Read the model definition and answer for the solid it produces. Units are mm, in the model's axes. A direction names the side the tool comes from. Give positions to 0.01 mm unless a question says otherwise; leave off trailing zeros. Loops run counter-clockwise (first coordinate to the right, second up) from the corner with the lowest first, then second, coordinate; pieces in that order, holes last. Notation, with made-up numbers: (25.5, 58.25) - (47.5, 58.25) arc R5 cw to (47.5, 62.25) - close; hole circle Ø4 at (14, 73). An arc over 180 degrees is marked (long way). Put each result on its own line as item: value. Start each with the question number.
1. A cutting plane is placed at A-A, the plane y = 10.5. Determine the outline of the cut face in (x, z) (3 decimals).
2. A cutting plane is placed at C-C, the plane x = 25.4. Determine the outline of the cut face in (y, z) (1 decimal), plus the area to 3 significant figures.
3. A cutting plane is placed at B-B, the plane z = 253.5. Determine the outline of the cut face in (x, y) (3 decimals), plus the area to 3 significant figures.
4. For faces 1 (the flat face through (25, 23, 0)), 2 (the cylindrical face through (22.3, 23.83, 536.71)), 3 (the flat face through (26, 22.225, 299)), determine the directions among +Z, -Z, +X, -X, +Y, -Y from which every point of the face is accessible in a straight line to the end or side of a thin tool.
5. Consider L1, parallel to X at y = 20, z = 333.5 (3 decimals); L2, parallel to Y at x = 37.5, z = 538 (3 decimals); L3, parallel to Z at x = 25.4, y = 23.2. Determine where each line is inside the solid, lowest interval first. Write a range as from..to.
6. A cutting plane is placed at D-D, the plane z = 25.4. Determine the outline of the cut face in (x, y) (1 decimal).
7. For a pull along Y with two mould halves and no side action, classify faces 4 (the flat face through (47.625, 13, 281)), 5 (the cylindrical face through (14.87, 23.835, 15.744)), 6 (the flat face through (25, 25.4, 301)) as released by +Y, released by -Y, zero draft, split by the parting line, or undercut.
8. Given pin 1 Ø2 at (x, y) = (7.5, 6) entering from -Z, flat-ended and moving along its own axis, determine where the tip first touches the part or whether it passes through.
```python
from build123d import *

# Parameters (mm, degrees)
SKETCH1_W           = 50.8
SKETCH1_H           = 25.4
BOSS_EXTRUDE1_DEPTH = 609.6
SKETCH2_W           = 44.45
SKETCH2_H           = 19.05
CUT_EXTRUDE1_DEPTH  = 609.6
CUT_EXTRUDE3_DEPTH  = 25.4
SKETCH6_R           = 14.2875
CUT_EXTRUDE5_DEPTH  = 3.175
SKETCH8_R           = 14.2875
CUT_EXTRUDE7_DEPTH  = 3.175


with BuildPart() as part:
    # Sketch1 → Boss-Extrude1 (new body)
    with BuildSketch(Plane.XY):
        with Locations((25.4, 12.7)):
            Rectangle(SKETCH1_W, SKETCH1_H)
    extrude(amount=BOSS_EXTRUDE1_DEPTH)

    # Sketch2 → Cut-Extrude1 (cut)
    with BuildSketch(Plane(origin=(0, 0, 0), x_dir=(-1, 0, 0), z_dir=(0, 0, -1))):
        with Locations((-25.4, 12.7)):
            Rectangle(SKETCH2_W, SKETCH2_H)
    extrude(amount=-CUT_EXTRUDE1_DEPTH, mode=Mode.SUBTRACT)

    # Sketch4 → Cut-Extrude3 (cut)
    with BuildSketch(Plane.XZ):
        Polygon((0, 609.6), (50.8, 566.973738736), (50.8, 609.6), align=None)
    extrude(amount=-CUT_EXTRUDE3_DEPTH, mode=Mode.SUBTRACT)

    # Sketch6 → Cut-Extrude5 (cut)
    with BuildSketch(Plane(origin=(0, 25.4, 0), x_dir=(1, 0, 0), z_dir=(0, 1, 0))):
        with Locations((25.4, -25.4)):
            Circle(SKETCH6_R)
    extrude(amount=-CUT_EXTRUDE5_DEPTH, mode=Mode.SUBTRACT)

    # Sketch8 → Cut-Extrude7 (cut)
    with BuildSketch(Plane(origin=(0, 25.4, 0), x_dir=(1, 0, 0), z_dir=(0, 1, 0))):
        with Locations((25.4, -522.762581257)):
            Circle(SKETCH8_R)
    extrude(amount=-CUT_EXTRUDE7_DEPTH, mode=Mode.SUBTRACT)


solid = part.part
```
Return value:
1. outline: (0, 0) - (3.175, 0) - (3.175, 606.936) - (0, 609.6) - close; (47.625, 0) - (50.8, 0) - (50.8, 566.974) - (47.625, 569.638) - close
2. outline: (0, 0) - (3.2, 0) - (3.2, 588.3) - (0, 588.3) - close; (22.2, 0) - (25.4, 0) - (25.4, 11.1) - (22.2, 11.1) - close; (22.2, 39.7) - (25.4, 39.7) - (25.4, 508.5) - (22.2, 508.5) - close; (22.2, 537.1) - (25.4, 537.1) - (25.4, 588.3) - (22.2, 588.3) - close
2. area: 3,550 mm2
3. outline: (0, 0) - (50.8, 0) - (50.8, 25.4) - (0, 25.4) - close; hole (3.175, 3.175) - (47.625, 3.175) - (47.625, 22.225) - (3.175, 22.225) - close
3. area: 444 mm2
4. face 1: -Z, +X, -X, +Y, -Y
4. face 2: +Y
4. face 3: +Z, -Z
5. L1: x = 0..3.175, 47.625..50.8
5. L2: y = 0..3.175, 22.225..25.4
5. L3: z = 0..11.11, 39.69..508.48, 537.05..588.29
6. outline: (0, 0) - (50.8, 0) - (50.8, 25.4) - (39.7, 25.4) - (39.7, 22.2) - (47.6, 22.2) - (47.6, 3.2) - (3.2, 3.2) - (3.2, 22.2) - (11.1, 22.2) - (11.1, 25.4) - (0, 25.4) - close
7. face 4: undercut
7. face 5: zero draft
7. face 6: released by +Y
8. pin 1: passes through
